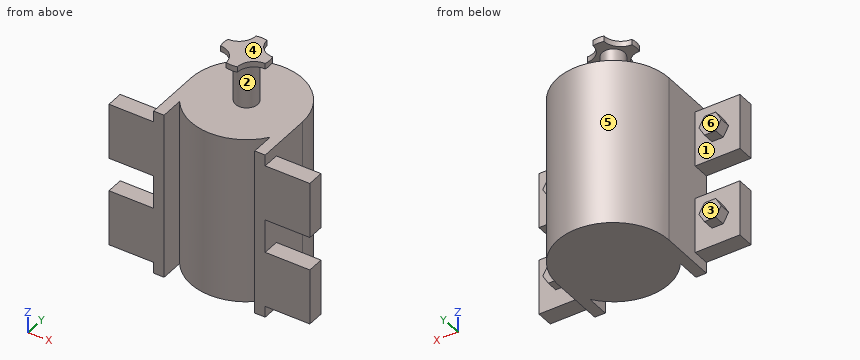
```python
from build123d import *

# Parameters (mm, degrees)
SZKIC1_R                    = 50
DODANIE_WYCI_GNI_CIE1_DEPTH = 150
SZKIC2_R                    = 10
DODANIE_WYCI_GNI_CIE2_DEPTH = 40
DODANIE_WYCI_GNI_CIE3_DEPTH = 5
DODANIE_WYCI_GNI_CIE4_DEPTH = 150
SZKIC5_W                    = 50
SZKIC5_H                    = 15
DODANIE_WYCI_GNI_CIE5_DEPTH = 40
DODANIE_WYCI_GNI_CIE6_DEPTH = 10


with BuildPart() as part:
    # Szkic1 → Dodanie-wyciągnięcie1 (new body)
    with BuildSketch(Plane.XY):
        Circle(SZKIC1_R)
    extrude(amount=DODANIE_WYCI_GNI_CIE1_DEPTH)

    # Szkic2 → Dodanie-wyciągnięcie2 (add)
    with BuildSketch(Plane.XY.offset(150)):
        Circle(SZKIC2_R)
    extrude(amount=DODANIE_WYCI_GNI_CIE2_DEPTH)

    # Szkic3 → Dodanie-wyciągnięcie3 (add)
    with BuildSketch(Plane.XY.offset(190)):
        with BuildLine():
            ThreePointArc((-5, -20), (-9.393398282, -9.393398282), (-20, -5))
            ThreePointArc((-20, -5), (-20.615528128, 0), (-20, 5))
            ThreePointArc((-20, 5), (-9.393398282, 9.393398282), (-5, 20))
            ThreePointArc((-5, 20), (0, 20.615528128), (5, 20))
            ThreePointArc((5, 20), (9.393398282, 9.393398282), (20, 5))
            ThreePointArc((20, 5), (20.615528128, 0), (20, -5))
            ThreePointArc((20, -5), (9.393398282, -9.393398282), (5, -20))
            ThreePointArc((5, -20), (0, -20.615528128), (-5, -20))
        make_face()
    extrude(amount=DODANIE_WYCI_GNI_CIE3_DEPTH)

    # Szkic4 → Dodanie-wyciągnięcie4 (add)
    with BuildSketch(Plane.XY):
        Polygon((-50, 0), (-50, -50), (-40.610421469, -50), (-40.610421469, -29.168367595), align=None)
    dodanie_wyci_gni_cie4 = extrude(amount=DODANIE_WYCI_GNI_CIE4_DEPTH)

    # Szkic5 → Dodanie-wyciągnięcie5 (add)
    with BuildSketch(Plane.ZY.offset(50)):
        with Locations((35, -42.5)):
            Rectangle(SZKIC5_W, SZKIC5_H)
        with Locations((115, -42.5)):
            Rectangle(SZKIC5_W, SZKIC5_H)
    dodanie_wyci_gni_cie5 = extrude(amount=DODANIE_WYCI_GNI_CIE5_DEPTH)

    # Szkic6 → Dodanie-wyciągnięcie6 (add)
    with BuildSketch(Plane(origin=(0, -35, 0), x_dir=(1, 0, 0), z_dir=(0, 1, 0))):
        Polygon((-65, -26.339745962), (-75, -26.339745962), (-80, -35), (-75, -43.660254038), (-65, -43.660254038), (-60, -35), align=None)
        Polygon((-60, -115), (-65, -106.339745962), (-75, -106.339745962), (-80, -115), (-75, -123.660254038), (-65, -123.660254038), align=None)
    dodanie_wyci_gni_cie6 = extrude(amount=DODANIE_WYCI_GNI_CIE6_DEPTH)

    # Lustro1: Dodanie-wyciągnięcie4, Dodanie-wyciągnięcie5, Dodanie-wyciągnięcie6 across plane
    add(dodanie_wyci_gni_cie4.mirror(Plane(origin=(0, 0, 0), x_dir=(0, 0, 1), z_dir=(1, 0, 0))))
    add(dodanie_wyci_gni_cie5.mirror(Plane(origin=(0, 0, 0), x_dir=(0, 0, 1), z_dir=(1, 0, 0))))
    add(dodanie_wyci_gni_cie6.mirror(Plane(origin=(0, 0, 0), x_dir=(0, 0, 1), z_dir=(1, 0, 0))))


solid = part.part
```
Part model, mm, in its own coordinate system. Face numbers are marked on the shaded views. A direction names the side the tool comes from. Give positions to 0.01 mm unless a question says otherwise; leave off trailing zeros. Write each loop counter-clockwise with the first axis right and the second up, starting at its lowest first coordinate (ties: lowest second). Pieces come first, ordered by that corner, then holes. Notation, with made-up numbers: (45, -11.75) -> (71, -11.75) arc R14 ccw to (71, 9.25) -> close; hole circle Ø6 at (-37, 57.5). An arc over 180 degrees is marked (long way). Put each result on its own line as item: value. Start each with the question number.
Item 1: Cut at B-B (z = 81.5). List the corners of the cut face in (x, y).
Item 2: Cut at D-D (x = -30.5). List the corners of the cut face in (y, z), then the cut area to 3 significant figures.
Item 3: Pull direction Z, two halves, no side cores. Call the marked faces 1, 2, 3 and 4: pulls with the +Z half, pulls with the -Z half, needs draft (parallel to the pull), parting line crosses it, or undercut.
Item 4: Which spindle directions (+Z, -Z, +X, -X, +Y, -Y) get a long thin tool onto all of the face, cutting with end or side? Do the marked faces 5 and 6. Say none if no direction does.
Item 5: Cut at A-A (x = 0). List the corners of the cut face in (y, z), then the cut area to 3 significant figures.
Item 6: Wall check: L1, parallel to X at y = -29.5, z = 12.5; L2, parallel to X at y = -37.5, z = 140.5; L3, parallel to Z at x = 38, y = -15. Give the ranges that are in metal, low to high. Write a range as [from, to].
Item 7: Pin check, flat tips, straight feed: pin 1 Ø8 at (x, y) = (72, -32) entering from -Z; pin 2 Ø5 at (x, z) = (68.5, 35.5) entering from +Y; pin 3 Ø1.5 at (x, y) = (37.5, 4) entering from +Z. Stop position of each tip, or through.
Item 8: Cut at C-C (y = -32). State how many separate pieces and enclosed holes the cut face has, then the cut area to 3 significant figures.
Answer list:
1. outline: (-50, -50) -> (-40.61, -50) -> (-40.61, -29.17) arc R50 ccw to (40.61, -29.17) -> (40.61, -50) -> (50, -50) -> (50, 0) arc R50 ccw to (-50, 0) -> close
2. outline: (-39.62, 0) -> (39.62, 0) -> (39.62, 150) -> (-39.62, 150) -> close
2. area: 11,900 mm2
3. face 1: undercut
3. face 2: undercut
3. face 3: needs draft
3. face 4: pulls with the +Z half
4. face 5: +Z, -Z, +Y
4. face 6: +Z, -Z, -X, +Y
5. outline: (-50, 0) -> (50, 0) -> (50, 150) -> (10, 150) -> (10, 190) -> (20.62, 190) -> (20.62, 195) -> (-20.62, 195) -> (-20.62, 190) -> (-10, 190) -> (-10, 150) -> (-50, 150) -> close
5. area: 16,000 mm2
6. L1: x = [-50, -40.61], [-40.37, 40.37], [40.61, 50]
6. L2: x = [-50, -40.61], [-33.07, 33.07], [40.61, 50]
6. L3: z = [0, 150]
7. pin 1: stops at z = 10
7. pin 2: stops at y = -25
7. pin 3: stops at z = 150
8. separate pieces: 7
8. enclosed holes: 0
8. area: 15,400 mm2
